from build123d import *

# Parameters (mm, degrees)
SKETCH_1_R      = 1.1
EXTRUDE_1_DEPTH = 5.6
EXTRUDE_2_DEPTH = 1.5


with BuildPart() as part:
    # 草图1 → 凸台-拉伸1 (new body)
    with BuildSketch(Plane.XY):
        Polygon((1.8, 0.4), (2.2, 0), (4, 0), (4.4, 0.4), (8.3, 0.4), (8.7, 0), (10.5, 0), (10.9, 0.4), (12.7, 0.4), (12.7, 6.5), (2.517906402, 6.5), (2, 6.5), (0, 6.5), (0, 0.4), align=None)
        with Locations((3.1, 1.5)):
            Circle(SKETCH_1_R, mode=Mode.SUBTRACT)
        with Locations((9.6, 1.5)):
            Circle(SKETCH_1_R, mode=Mode.SUBTRACT)
    extrude(amount=EXTRUDE_1_DEPTH)

    # 草图3 → 凸台-拉伸2 (add, symmetric)
    with BuildSketch(Plane.XY.offset(2.8)):
        Polygon((1.8, 6.5), (13.7, 13.5), (13.84831969, 13.247856527), (2.238287657, 6.5), align=None)
    extrude(amount=EXTRUDE_2_DEPTH, both=True)


solid = part.part
For this review, take the finished solid that the model builds, in its own axes (mm). A direction names the side the tool comes from. Round coordinates to 2 decimals unless told otherwise and drop trailing zeros. Loops run counter-clockwise (first coordinate to the right, second up) from the corner with the lowest first, then second, coordinate; pieces in that order, holes last. Notation, with made-up numbers: (84, 5.25) - (114, 5.25) arc R25 cw to (114, 27.25) - close; hole circle Ø10 at (38, 60). An arc over 180 degrees is marked (long way). Use one line per item in the form item = value.
Item 1: Consider section B-B on z = 4.5. Write out the cut boundary in (x, y), then the cut area to 3 significant figures.
Answers:
outline = (0, 0.4) - (1.8, 0.4) - (2.2, 0) - (4, 0) - (4.4, 0.4) - (8.3, 0.4) - (8.7, 0) - (10.5, 0) - (10.9, 0.4) - (12.7, 0.4) - (12.7, 6.5) - (0, 6.5) - close; hole circle Ø2.2 at (3.1, 1.5); hole circle Ø2.2 at (9.6, 1.5)
area = 71.6 mm^2
Item 2: For line 1 (X direction, y = 1.25, z = 5.1); line 2 (X direction, y = 2.5, z = 1.15); line 3 (X direction, y = 4, z = 3.35), list the stretches that pass through material, from the lowest coordinate up.
Answers:
line_1 = 0 to 2.03, 4.17 to 8.53, 10.67 to 12.7
line_2 = 0 to 2.64, 3.56 to 9.14, 10.06 to 12.7
line_3 = 0 to 12.7
Item 3: Consider section D-D on z = 3.3. Write out the cut boundary in (x, y).
Answers:
outline = (0, 0.4) - (1.8, 0.4) - (2.2, 0) - (4, 0) - (4.4, 0.4) - (8.3, 0.4) - (8.7, 0) - (10.5, 0) - (10.9, 0.4) - (12.7, 0.4) - (12.7, 6.5) - (2.24, 6.5) - (13.85, 13.25) - (13.7, 13.5) - (1.8, 6.5) - (0, 6.5) - close; hole circle Ø2.2 at (3.1, 1.5); hole circle Ø2.2 at (9.6, 1.5)
Item 4: Clearance check with flat-ended pins moving along their axes: P1, Ø0.9, axis at x = 1, z = 2.5, coming from the -Y side; P2, Ø2, axis at x = 6.5, y = 8.5, coming from the -Z side; P3, Ø4, axis at x = 9, y = 10, coming from the +Z side. State where each tip first meets the part, or that it passes through.
Answers:
P1 = 0.4
P2 = 1.3
P3 = 4.3
Item 5: Consider section A-A on y = 1.5. Write out the cut boundary in (x, z), then the cut area to 3 significant figures.
Answers:
outline = (0, 0) - (2, 0) - (2, 5.6) - (0, 5.6) - close; (4.2, 0) - (8.5, 0) - (8.5, 5.6) - (4.2, 5.6) - close; (10.7, 0) - (12.7, 0) - (12.7, 5.6) - (10.7, 5.6) - close
area = 46.5 mm^2
Item 6: Consider section C-C on x = 7.75. Write out the cut boundary in (y, z), then the cut area to 3 significant figures.
Answers:
outline = (0.4, 0) - (6.5, 0) - (6.5, 5.6) - (0.4, 5.6) - close; (9.7, 1.3) - (10, 1.3) - (10, 4.3) - (9.7, 4.3) - close
area = 35.0 mm^2
Item 7: Mouldability with a two-part tool opening along Y and no side actions: class faces 1 (the cylindrical face through (3.69, 2.43, 2.76)), 2 (the flat face through (12, 0.4, 3)), 3 (the flat face through (6, 3, 0)) as +Y half, -Y half, draft (parallel to the pull), parting line (faces both ways), or undercut.
Answers:
face_1 = undercut
face_2 = -Y half
face_3 = draft
Item 8: Tool access review of faces 4 (the flat face through (1, 0.4, 3)), 5 (the flat face through (8.12, 9.92, 2.82)), 6 (the flat face through (6, 0.4, 3)): name each direction out of +Z, -Z, +X, -X, +Y, -Y from which nothing blocks a thin tool from reaching the whole face with its end or side.
Answers:
face_4 = +Z, -Z, -X, -Y
face_5 = +Z, -Z, +X
face_6 = +Z, -Z, -Y
